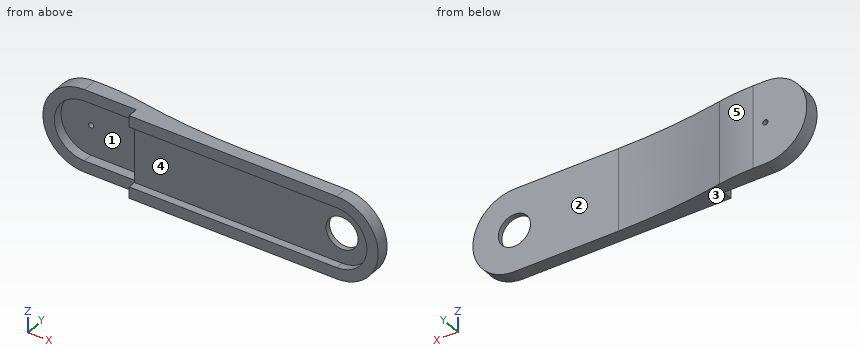
```python
from build123d import *

# Parameters (mm, degrees)
BOSS_EXTRUDE1_DEPTH     = 7.5
CUT_EXTRUDE1_DEPTH      = 293.841680776
CUT_EXTRUDE1_DEPTH_BACK = 293.841680776
BOSS_EXTRUDE3_DEPTH     = 5
CUT_EXTRUDE2_DEPTH      = 293.841680776
CUT_EXTRUDE2_DEPTH_BACK = 293.841680776
SKETCH11_R              = 15.5
SKETCH12_W              = 30
SKETCH12_H              = 11
SKETCH12_H_2            = 58
BOSS_EXTRUDE4_DEPTH     = 7
BOSS_EXTRUDE5_DEPTH     = 5
BOSS_EXTRUDE6_START     = 2.5
BOSS_EXTRUDE6_DEPTH     = 2.5
CUT_EXTRUDE3_DEPTH      = 294.394359182
CUT_EXTRUDE3_DEPTH_BACK = 294.394359182
SKETCH15_R              = 2.5
FILLET1_R               = 200
FILLET2_R               = 600


with BuildPart() as part:
    # Sketch1 → Boss-Extrude1 (new body)
    with BuildSketch(Plane(origin=(0, 0, 0), x_dir=(1, 0, 0), z_dir=(0, 1, 0))):
        with BuildLine():
            Line((0, -40), (250, -40))
            ThreePointArc((250, -40), (290, 0), (250, 40))
            Line((250, 40), (0, 40))
            ThreePointArc((0, 40), (-40, 0), (0, -40))
        make_face()
        with BuildLine():
            Line((0, 29), (250, 29))
            ThreePointArc((250, 29), (279, 0), (250, -29))
            Line((250, -29), (0, -29))
            ThreePointArc((0, -29), (-29, 0), (0, 29))
        make_face(mode=Mode.SUBTRACT)
    extrude(amount=BOSS_EXTRUDE1_DEPTH)

    # Sketch9 → Cut-Extrude1 (cut, two sides: drawn at the far end of the back side and taken through both)
    with BuildSketch(Plane(origin=(0, 7.5, 0), x_dir=(1, 0, 0), z_dir=(0, 1, 0)).offset(-CUT_EXTRUDE1_DEPTH_BACK)):
        with BuildLine():
            Line((50, 29), (50, -29))
            Line((50, -29), (250, -29))
            ThreePointArc((250, -29), (279, 0), (250, 29))
            Line((250, 29), (50, 29))
        make_face()
        with BuildLine():
            Line((0, -40), (50, -40))
            Line((50, -40), (50, -29))
            Line((50, -29), (0, -29))
            ThreePointArc((0, -29), (-29, 0), (0, 29))
            Line((0, 29), (50, 29))
            Line((50, 29), (50, 40))
            Line((50, 40), (0, 40))
            ThreePointArc((0, 40), (-40, 0), (0, -40))
        make_face()
    extrude(amount=CUT_EXTRUDE1_DEPTH + CUT_EXTRUDE1_DEPTH_BACK, mode=Mode.SUBTRACT)

    # Sketch9<3> → Boss-Extrude3 (add)
    with BuildSketch(Plane(origin=(0, 7.5, 0), x_dir=(1, 0, 0), z_dir=(0, 1, 0))):
        with BuildLine():
            Line((50, 40), (50, -40))
            Line((50, -40), (250, -40))
            ThreePointArc((250, -40), (290, 0), (250, 40))
            Line((250, 40), (50, 40))
        make_face()
    extrude(amount=BOSS_EXTRUDE3_DEPTH)

    # Sketch11 → Cut-Extrude2 (cut, two sides: drawn at the far end of the back side and taken through both)
    with BuildSketch(Plane.XZ.offset(-7.5).offset(-CUT_EXTRUDE2_DEPTH_BACK)):
        with Locations(Location((250, 0, 0), (0, 0, 270))):
            Circle(SKETCH11_R)
    extrude(amount=CUT_EXTRUDE2_DEPTH + CUT_EXTRUDE2_DEPTH_BACK, mode=Mode.SUBTRACT)

    # Sketch12 → Boss-Extrude4 (add)
    with BuildSketch(Plane(origin=(0, 12.5, 0), x_dir=(1, 0, 0), z_dir=(0, 1, 0))):
        with Locations((65, -34.5)):
            Rectangle(SKETCH12_W, SKETCH12_H)
        with BuildLine():
            ThreePointArc((0, 40), (-40, 0), (0, -40))
            Line((0, -40), (50, -40))
            Line((50, -40), (50, -29))
            Line((50, -29), (0, -29))
            ThreePointArc((0, -29), (-29, 0), (0, 29))
            Line((0, 29), (50, 29))
            Line((50, 29), (50, 40))
            Line((50, 40), (0, 40))
        make_face()
        with Locations((65, 34.5)):
            Rectangle(SKETCH12_W, SKETCH12_H)
        with Locations((65, 0)):
            Rectangle(SKETCH12_W, SKETCH12_H_2)
    extrude(amount=BOSS_EXTRUDE4_DEPTH)

    # Sketch13 → Boss-Extrude5 (add)
    with BuildSketch(Plane(origin=(0, 19.5, 0), x_dir=(1, 0, 0), z_dir=(0, 1, 0))):
        with BuildLine():
            Line((80, -40), (80, 40))
            Line((80, 40), (0, 40))
            ThreePointArc((0, 40), (-40, 0), (0, -40))
            Line((0, -40), (80, -40))
        make_face()
    extrude(amount=BOSS_EXTRUDE5_DEPTH)

    # Sketch14 → Boss-Extrude6 (add)
    with BuildSketch(Plane.XZ.offset(-12.5).offset(BOSS_EXTRUDE6_START)):
        with BuildLine():
            Line((0, -40), (50, -40))
            Line((50, -40), (50, -29))
            Line((50, -29), (0, -29))
            ThreePointArc((0, -29), (-29, 0), (0, 29))
            Line((0, 29), (50, 29))
            Line((50, 29), (50, 40))
            Line((50, 40), (0, 40))
            ThreePointArc((0, 40), (-40, 0), (0, -40))
        make_face()
    extrude(amount=-BOSS_EXTRUDE6_DEPTH)

    # Sketch15 → Cut-Extrude3 (cut, two sides: drawn at the far end of the back side and taken through both)
    with BuildSketch(Plane.XZ.offset(-19.5).offset(-CUT_EXTRUDE3_DEPTH_BACK)):
        with Locations(Location((0, 0, 0), (0, 0, 270))):
            Circle(SKETCH15_R)
    extrude(amount=CUT_EXTRUDE3_DEPTH + CUT_EXTRUDE3_DEPTH_BACK, mode=Mode.SUBTRACT)

    # Fillet1
    # the kernel refuses this fillet: 200 mm, written as the material it takes off along each edge
    with BuildSketch(Plane(origin=(80, 24.5, 210.587221092), x_dir=(0, -1, 0), z_dir=(0, 0, -1))) as fillet1_piece_1:
        with BuildLine():
            CenterArc((200, 68.234888437), FILLET1_R, 180, 19.948443589)
            Line((0, 68.234888437), (-4, 68.234888437))
            Line((-4, 68.234888437), (-4, 0))
            Line((-4, 0), (0, -4))
            ThreePointArc((0, -4), (6, -4), (8.24, -1.364697769))
            Line((8.24, -1.364697769), (12, 0))
        make_face()
    extrude(amount=421.174442185, mode=Mode.SUBTRACT)

    # Fillet2
    fillet2_edges = [part.edges().sort_by_distance(p)[0] for p in [
        (80, 12.5, 0),
    ]]
    fillet(fillet2_edges, radius=FILLET2_R)


solid = part.part
```
Here's how the part is built. I have some questions about the finished solid (model axes, mm). Face numbers are marked on the shaded views. A direction names the side the tool comes from. Give positions to 0.01 mm unless a question says otherwise; leave off trailing zeros. Order: outer loops, then holes, each group sorted by start corner. A loop starts at its lowest first (then second) coordinate and runs counter-clockwise, first axis right, second up. Notation, with made-up numbers: (-9.5, -26.75) -> (36.5, -26.75) arc R35 ccw to (36.5, 6.25) -> close; hole circle Ø3 at (52, 30). An arc over 180 degrees is marked (long way). Use CSV: the item, a comma, the result in double quotes. Start each with the question number.
Item 1: Suppose I cut it at C-C (z = -23.5). List the corners of the cut face in (x, y) for me, and give its area (3 significant figures).
Item 2: Suppose I cut it at B-B (x = 260). List the corners of the cut face in (y, z) for me.
Item 3: Thinking about a two-plate mould opening in Z: for the marked faces 1, 2 and 3, which applies, pulls with the +Z half, pulls with the -Z half, needs draft (parallel to the pull), parting line crosses it, or undercut?
Item 4: I'm going to push flat-ended pins straight in: P1, Ø8, axis at y = 13.5, z = -6.5, coming from the +X side; P2, Ø5, axis at x = 152, z = 26, coming from the -Y side; P3, Ø12, axis at y = 17, z = 26, coming from the +X side. Where does each tip first touch, or does it pass through?
Item 5: If I drill on probe 1 along X at (y, z) = (11.1, 0); probe 2 along Z at (x, y) = (163, 7); probe 3 along Z at (x, y) = (250, 10.45), over which ranges is the centre line in solid material (lowest first)? Write a range as [from, to].
Item 6: On a 3-axis mill with a long thin cutter (end or side, diameter ignored), from which of +Z, -Z, +X, -X, +Y, -Y can I reach the whole of each face in a straight line? I mean the marked faces 4 and 5. Say none if no direction works.
Item 7: Suppose I cut it at A-A (y = 4.75). List the corners of the cut face in (x, z) for me.
Item 8: Suppose I cut it at D-D (x = 224). List the corners of the cut face in (y, z) for me.
Answer block:
1,outline,"(-32.37, 10) -> (-16.99, 10) -> (-16.99, 19.5) -> (50, 19.5) -> (50, 7.5) -> (266.99, 7.5) -> (266.99, 0) -> (282.37, 0) -> (282.37, 12.5) -> (149.81, 12.5) arc R600 cw to (46.28, 21.5) arc R200 ccw to (11.77, 24.5) -> (-32.37, 24.5) -> close"
1,area,"2,070 mm^2"
2,outline,"(0, -38.73) -> (12.5, -38.73) -> (12.5, -11.84) -> (7.5, -11.84) -> (7.5, -27.22) -> (0, -27.22) -> close; (0, 27.22) -> (7.5, 27.22) -> (7.5, 11.84) -> (12.5, 11.84) -> (12.5, 38.73) -> (0, 38.73) -> close"
3,face 1,"undercut"
3,face 2,"needs draft"
3,face 3,"pulls with the -Z half"
4,P1,"stops at x = 289.91"
4,P2,"stops at y = 7.5"
4,P3,"stops at x = 283.39"
5,probe 1,"x = [-40, -29], [50, 234.5], [265.5, 290]"
5,probe 2,"z = [-40, -29], [29, 40]"
5,probe 3,"z = [-40, -15.5], [15.5, 40]"
6,face 4,"-X, -Y"
6,face 5,"+Z, -Z, +X, +Y"
7,outline,"(50, -40) -> (250, -40) arc R40 ccw to (250, 40) -> (50, 40) -> (50, 29) -> (250, 29) arc R29 cw to (250, -29) -> (50, -29) -> close"
8,outline,"(0, -40) -> (12.5, -40) -> (12.5, 40) -> (0, 40) -> (0, 29) -> (7.5, 29) -> (7.5, -29) -> (0, -29) -> close"
